```python
from build123d import *

# Parameters (mm, degrees)
SKETCH1_W           = 239.395
SKETCH1_H           = 55.245
SKETCH1_W_2         = 231.775
SKETCH1_H_2         = 47.625
BOSS_EXTRUDE1_DEPTH = 23.876
SKETCH2_W           = 27.501576043
SKETCH2_H           = 47.625
SKETCH2_W_2         = 27.249268006
SKETCH2_H_2         = 3.81
SKETCH2_W_3         = 25.735419783
SKETCH2_H_3         = 55.245
BOSS_EXTRUDE2_DEPTH = 3.81
SKETCH3_W           = 12.907242676
SKETCH3_H           = 13.858802321
CUT_EXTRUDE1_DEPTH  = 3.81
SKETCH4_R           = 2.38125
BOSS_EXTRUDE3_DEPTH = 3.81


with BuildPart() as part:
    # Sketch1 → Boss-Extrude1 (new body)
    with BuildSketch(Plane(origin=(0, 0, 0), x_dir=(1, 0, 0), z_dir=(0, 1, 0))):
        with Locations((62.882734648, -14.00661841)):
            Rectangle(SKETCH1_W, SKETCH1_H)
        with Locations((62.882734648, -14.00661841)):
            Rectangle(SKETCH1_W_2, SKETCH1_H_2, mode=Mode.SUBTRACT)
    extrude(amount=BOSS_EXTRUDE1_DEPTH)

    # Sketch2 → Boss-Extrude2 (add)
    with BuildSketch(Plane.XZ):
        with Locations((0.436495468, 14.00661841)):
            Rectangle(SKETCH2_W, SKETCH2_H)
        with Locations((122.427431402, 14.00661841)):
            Rectangle(SKETCH2_W_2, SKETCH2_H)
        with Locations((122.427431402, 39.72411841)):
            Rectangle(SKETCH2_W_2, SKETCH2_H_2)
        with Locations((0.436495468, 39.72411841)):
            Rectangle(SKETCH2_W, SKETCH2_H_2)
        with Locations((0.436495468, -11.71088159)):
            Rectangle(SKETCH2_W, SKETCH2_H_2)
        with Locations((122.427431402, -11.71088159)):
            Rectangle(SKETCH2_W_2, SKETCH2_H_2)
        with Locations((63.135042686, 14.00661841)):
            Rectangle(SKETCH2_W_3, SKETCH2_H_3)
    extrude(amount=BOSS_EXTRUDE2_DEPTH)

    # Sketch3 → Cut-Extrude1 (cut)
    with BuildSketch(Plane.ZY.offset(56.814765352)):
        with Locations((30.592232843, 6.929401161)):
            Rectangle(SKETCH3_W, SKETCH3_H)
    extrude(amount=-CUT_EXTRUDE1_DEPTH, mode=Mode.SUBTRACT)

    # Sketch4 → Boss-Extrude3 (add)
    # profile 1 of 4: a face of its own
    with BuildSketch(Plane(origin=(0, 23.876, 0), x_dir=(1, 0, 0), z_dir=(0, 1, 0))):
        with BuildLine():
            Line((-10.412074004, 13.61588159), (5.743340555, 13.61588159))
            ThreePointArc((5.743340555, 13.61588159), (-2.334366725, 23.314823136), (-10.412074004, 13.61588159))
        make_face()
        with Locations(Location((-2.334366725, 17.917758685, 0), (0, 0, 270))):
            Circle(SKETCH4_R, mode=Mode.SUBTRACT)
    # profile 2 of 4: a face of its own
    with BuildSketch(Plane(origin=(0, 23.876, 0), x_dir=(1, 0, 0), z_dir=(0, 1, 0))):
        with BuildLine():
            Line((-10.412074004, -41.62911841), (5.743340555, -41.62911841))
            ThreePointArc((5.743340555, -41.62911841), (-2.334366725, -51.744975779), (-10.412074004, -41.62911841))
        make_face()
        with Locations(Location((-2.334366725, -45.991983403, 0), (0, 0, 270))):
            Circle(SKETCH4_R, mode=Mode.SUBTRACT)
    # profile 3 of 4: a face of its own
    with BuildSketch(Plane(origin=(0, 23.876, 0), x_dir=(1, 0, 0), z_dir=(0, 1, 0))):
        with BuildLine():
            Line((119.805130889, -41.62911841), (137.369914175, -41.62911841))
            ThreePointArc((137.369914175, -41.62911841), (128.587522532, -52.012034088), (119.805130889, -41.62911841))
        make_face()
        with Locations(Location((128.587522532, -45.991983403, 0), (0, 0, 270))):
            Circle(SKETCH4_R, mode=Mode.SUBTRACT)
    # profile 4 of 4: a face of its own
    with BuildSketch(Plane(origin=(0, 23.876, 0), x_dir=(1, 0, 0), z_dir=(0, 1, 0))):
        with BuildLine():
            Line((119.805130889, 13.61588159), (137.369914175, 13.61588159))
            ThreePointArc((137.369914175, 13.61588159), (128.587522532, 23.697328425), (119.805130889, 13.61588159))
        make_face()
        with Locations(Location((128.587522532, 17.917758685, 0), (0, 0, 270))):
            Circle(SKETCH4_R, mode=Mode.SUBTRACT)
    extrude(amount=-BOSS_EXTRUDE3_DEPTH)


solid = part.part
```
For this review, take the finished solid that the model builds, in its own axes (mm). A direction names the side the tool comes from. Give positions to 0.01 mm unless a question says otherwise; leave off trailing zeros. Write each loop counter-clockwise with the first axis right and the second up, starting at its lowest first coordinate (ties: lowest second). Pieces come first, ordered by that corner, then holes. Notation, with made-up numbers: M 42.25,-5 L 50.25,-5 A34 cw 50.25,26 Z; hole C 69,-17 d4. An arc over 180 degrees is marked long. Answer as a JSON object with one key per item and string values. Group by question number.
Item 1: Draft analysis for pull direction Z (two halves, no side actions). For faces 5 (the flat face through (126, 20.066, -16)), 6 (the flat face through (0, 0, 14)), state which applies: +Z half, -Z half, draft (parallel to the pull), parting line (faces both ways), or undercut.
Item 2: Consider section A-A on z = 8. Write out the cut boundary in (x, y).
Item 3: For pin 1 Ø8.5 at (x, z) = (6.5, 15) entering from +Y; pin 2 Ø4 at (x, z) = (100, -11) entering from -Y; pin 3 Ø1.1 at (x, y) = (-54.5, 8) entering from +Z, all flat-tipped, find the tip position at first contact; note any pin that passes through.
Item 4: Consider section B-B on y = 16.25. Write out the cut boundary in (x, z).
Item 5: Consider section C-C on x = 87. Write out the cut boundary in (y, z), plus the area to 3 significant figures.
Item 6: Consider section D-D on y = 6.75. Write out the cut boundary in (x, z).
Item 7: For probe 1 along Z at (x, y) = (102.5, 9.25); probe 2 along X at (y, z) = (20.25, 9); probe 3 along Z at (x, y) = (-8, 20.75), list the stretches that pass through material, from the lowest coordinate up. Write a range as [from, to].
Item 8: Tool access review of faces 1 (the flat face through (-55, 7, 37.046)), 2 (the flat face through (136.052, -2, 14)), 3 (the flat face through (122, 0, 14)), 4 (the flat face through (32, 0, 40)): name each direction out of +Z, -Z, +X, -X, +Y, -Y from which nothing blocks a thin tool from reaching the whole face with its end or side.
Check result:
{
 "1": {"face 5": "draft", "face 6": "undercut"},
 "2": {"outline": "M -56.81,0 L -53,0 L -53,23.88 L -56.81,23.88 Z; M -13.31,-3.81 L 14.19,-3.81 L 14.19,0 L -13.31,0 Z; M 50.27,-3.81 L 76,-3.81 L 76,0 L 50.27,0 Z; M 108.8,-3.81 L 136.05,-3.81 L 136.05,0 L 108.8,0 Z; M 178.77,0 L 182.58,0 L 182.58,23.88 L 178.77,23.88 Z"},
 "3": {"pin 1": "stops at y = 0", "pin 2": "stops at y = 0", "pin 3": "stops at z = 41.63"},
 "4": {"outline": "M -56.81,-13.62 L 182.58,-13.62 L 182.58,41.63 L -56.81,41.63 Z; hole M -53,-9.81 L 178.77,-9.81 L 178.77,37.82 L -53,37.82 Z"},
 "5": {"outline": "M 0,-13.62 L 23.88,-13.62 L 23.88,-9.81 L 0,-9.81 Z; M 0,37.82 L 23.88,37.82 L 23.88,41.63 L 0,41.63 Z", "area": "182 mm^2"},
 "6": {"outline": "M -56.81,-13.62 L 182.58,-13.62 L 182.58,41.63 L -56.81,41.63 L -56.81,37.05 L -53,37.05 L -53,37.82 L 178.77,37.82 L 178.77,-9.81 L -53,-9.81 L -53,24.14 L -56.81,24.14 Z"},
 "7": {"probe 1": "z = [-13.62, -9.81], [37.82, 41.63]", "probe 2": "x = [-56.81, -53], [178.77, 182.58]", "probe 3": "z = [-21.05, -9.81], [37.82, 49.5]"},
 "8": {"face 1": "-X, -Y", "face 2": "+Z, -Z, +X, -Y", "face 3": "+Y", "face 4": "+Z, -Z, -Y"}
}
